Source: CAD feature listing. Evaluate the final solid. Frame: model axes, mm. A direction names the side the tool comes from. Round coordinates to 2 decimals unless told otherwise and drop trailing zeros. Loops run counter-clockwise (first coordinate to the right, second up) from the corner with the lowest first, then second, coordinate; pieces in that order, holes last. Notation, with made-up numbers: (27, 29.5) - (56, 29.5) arc R22 ccw to (56, 67.5) - close; hole circle Ø5 at (6, 35.25). An arc over 180 degrees is marked (long way). Use CSV: the item, a comma, the result in double quotes. Start each with the question number.
from build123d import *

# Parameters (mm, degrees)
SKETCH1_W              = 18
SKETCH1_H              = 80
BOSS_EXTRUDE1_DEPTH    = 46
BOSS_EXTRUDE2_DEPTH    = 27
BOSS_EXTRUDE3_START    = 33
SKETCH1_4_R            = 30
SKETCH1_4_R_2          = 18
BOSS_EXTRUDE3_DEPTH    = 24
FILLET1_R              = 16
BOSS_EXTRUDE4_DEPTH    = 6
BOSS_EXTRUDE5_DEPTH    = 9
F_16_0MM_DOWEL_HOLE1_D = 16
SKETCH3_W              = 48
SKETCH3_H              = 18
CUT_EXTRUDE1_DEPTH     = 88


with BuildPart() as part:
    # Sketch1 → Boss-Extrude1 (new, symmetric)
    with BuildSketch(Plane.XY):
        with Locations((-131, 30)):
            Rectangle(SKETCH1_W, SKETCH1_H)
    extrude(amount=BOSS_EXTRUDE1_DEPTH, both=True)

    # Sketch1_3 → Boss-Extrude2 (add, symmetric)
    with BuildSketch(Plane.XY):
        with BuildLine():
            ThreePointArc((0, -30), (-30, 0), (0, 30))
            Line((0, 30), (-82, 30))
            Line((-82, 30), (-82, 36))
            Line((-82, 36), (-122, 36))
            Line((-122, 36), (-122, -10))
            Line((-122, -10), (-104, -10))
            Line((-104, -10), (-104, 18))
            Line((-104, 18), (-44, 18))
            Line((-44, 18), (-44, -30))
            Line((-44, -30), (0, -30))
        make_face()
    extrude(amount=BOSS_EXTRUDE2_DEPTH, both=True)

    # Sketch1_4 → Boss-Extrude3 (add)
    with BuildSketch(Plane.XY.offset(BOSS_EXTRUDE3_START)):
        with Locations(Location((0, 0, 0), (0, 0, 90))):
            Circle(SKETCH1_4_R)
        Circle(SKETCH1_4_R_2, mode=Mode.SUBTRACT)
    boss_extrude3 = extrude(amount=-BOSS_EXTRUDE3_DEPTH)

    # Mirror1: Boss-Extrude3 across plane
    add(boss_extrude3.mirror(Plane.XY))

    # Fillet1
    fillet1_edges = [part.edges().sort_by_distance(p)[0] for p in [
        (-131, 70, 46),
        (-131, 70, -46),
    ]]
    fillet(fillet1_edges, radius=FILLET1_R)

    # Sketch1_7 → Boss-Extrude4 (add, symmetric)
    with BuildSketch(Plane.XY):
        Polygon((-122, 36), (-82, 36), (-122, 70), align=None)
    extrude(amount=BOSS_EXTRUDE4_DEPTH, both=True)

    # Sketch1_8 → Boss-Extrude5 (add, symmetric)
    with BuildSketch(Plane.XY):
        Polygon((-44, 18), (-44, -30), (-104, -10), (-104, 18), align=None)
    extrude(amount=BOSS_EXTRUDE5_DEPTH, both=True)

    # 16.0mm Dowel Hole1 (through all)
    with Locations(Plane(origin=(-122, 54, 30), x_dir=(0, 1, 0), z_dir=(1, 0, 0))):
        with Locations((0, 0), (0, -60)):
            Hole(F_16_0MM_DOWEL_HOLE1_D / 2)

    # Sketch3 → Cut-Extrude1 (cut)
    with BuildSketch(Plane(origin=(0, 30, 0), x_dir=(1, 0, 0), z_dir=(0, 1, 0))):
        Rectangle(SKETCH3_W, SKETCH3_H)
    extrude(amount=-CUT_EXTRUDE1_DEPTH, mode=Mode.SUBTRACT)


solid = part.part
1. Section query D-D on x = -116. Return the cut outline in (y, z).
2. Line query: line 1 along Z through (x, y) = (-133.25, 54); line 2 along Y through (x, z) = (0, -22.25); line 3 along X through (y, z) = (-1, 17). Output: solid intervals per line, ascending.
3. Reachability of faces 5 (the flat face through (-24, 24, 0)), 6 (the flat face through (-74, 0, 9)), 7 (the flat face through (-102, 36, -16)) from +Z, -Z, +X, -X, +Y, -Y: full face, straight path, thin tool, end or side. Return the list, or none.
4. Contact query for flat-ended pins moving along their axis: P1, Ø24, axis at x = -83, y = 2, coming from the +Z side; P2, Ø17, axis at x = -111, z = -17, coming from the +Y side; P3, Ø8, axis at y = -15.5, z = 11.5, coming from the +X side. Output: stop coordinate, or through.
5. Mould query, pull axis X, two halves, no side actions, for faces 1 (the flat face through (-24, -24, 0)), 2 (the flat face through (-74, 0, -9)), 3 (the flat face through (13, 13, 33)), 4 (the flat face through (-44, -6, 18)). Classes: +X half, -X half, draft (parallel to the pull), parting line (faces both ways), or undercut.
6. Section query B-B on x = -26.5. Return the cut outline in (y, z), and give its area (3 significant figures).
7. Section query C-C on z = 1. Return the cut outline in (x, y), and give its area (3 significant figures).
8. Section query A-A on y = 0. Give the number of separate pieces and of enclosed holes in the cut face, and give its area (3 significant figures).
Values:
1,outline,"(-10, -27) - (36, -27) - (36, -6) - (64.9, -6) - (64.9, 6) - (36, 6) - (36, 27) - (-10, 27) - close"
2,line 1,"z = -46 to -38, -22 to 22, 38 to 46"
2,line 2,"y = -30 to -18, 18 to 30"
2,line 3,"x = -140 to -104, -44 to -17.97, 17.97 to 29.98"
3,face 5,"+X, +Y, -Y"
3,face 6,"+Z, -Y"
3,face 7,"-Z, +X, +Y"
4,P1,"stops at z = 9"
4,P2,"stops at y = 36"
4,P3,"stops at x = 27.71"
5,face 1,"+X half"
5,face 2,"undercut"
5,face 3,"draft"
5,face 4,"undercut"
6,outline,"(-30, -27) - (-14.06, -27) - (-14.06, -33) - (14.06, -33) - (14.06, -27) - (30, -27) - (30, 27) - (14.06, 27) - (14.06, 33) - (-14.06, 33) - (-14.06, 27) - (-30, 27) - close; hole (-14.06, -9) - (14.06, -9) - (14.06, 9) - (-14.06, 9) - close"
6,area,"3,070 mm^2"
7,outline,"(-140, -10) - (-104, -10) - (-44, -30) - (-24, -30) - (-24, -18) arc R30 cw to (-24, 18) - (-24, 30) - (-82, 30) - (-82, 36) - (-122, 70) - (-140, 70) - close"
7,area,"7,130 mm^2"
8,separate pieces,"3"
8,enclosed holes,"0"
8,area,"5,620 mm^2"
